Design review of the part shown in the three views and the two pictorial views. Dimensions are in mm from the part's minimum x, y and z. Round coordinates to 2 decimals unless told otherwise and drop trailing zeros. Loops run counter-clockwise (first coordinate to the right, second up) from the corner with the lowest first, then second, coordinate; pieces in that order, holes last. Notation, with made-up numbers: (49, 15) - (86, 15) arc R11 cw to (86, 36) - close; hole circle Ø3 at (74.25, 47.25). An arc over 180 degrees is marked (long way). Return JSON: item names as keys, results as strings. Group by question number.
(1) We need section B-B, the plane x = 60. Write out the cut boundary in (y, z), and give its area (3 significant figures).
(2) We need section A-A, the plane y = 40. Write out the cut boundary in (x, z), and give its area (3 significant figures).
(3) Clearance check with flat-ended pins moving along their axes: pin 1 (4 mm diameter, centred on x = 85, z = 309, fed in from +Y); pin 2 (12 mm diameter, centred on x = 85.5, z = 232.5, fed in from -Y); pin 3 (1.5 mm diameter, centred on y = 66.5, z = 629, fed in from +X). State where each tip first meets the part, or that it passes through.
(4) Wall thickness on L1, parallel to Z at x = 23, y = 36; L2, parallel to X at y = 38, z = 379; L3, parallel to X at y = 53, z = 588.5: over which ranges is each line inside the solid? List them lowest first. Write a range as [from, to].
(5) We need section C-C, the plane z = 817.5. Write out the cut boundary in (x, y).
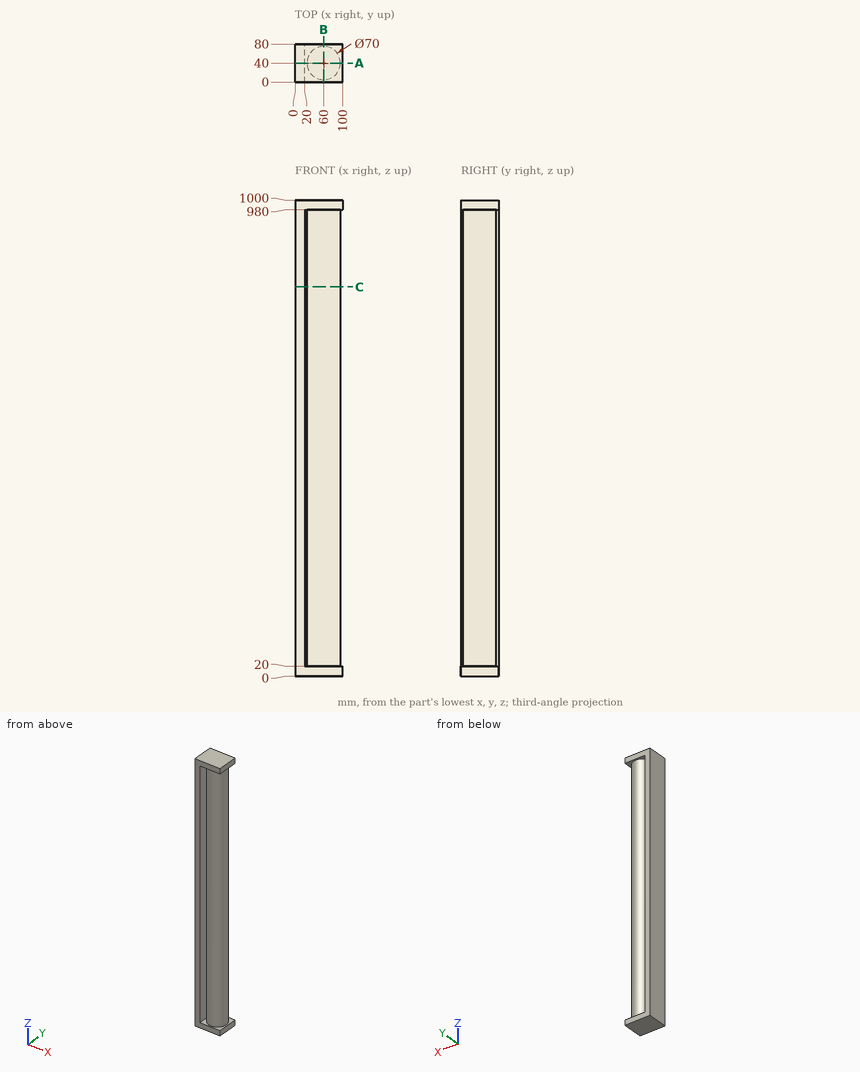
Solutions:
{
 "1": {"outline": "(0, 0) - (80, 0) - (80, 20) - (75, 20) - (75, 980) - (80, 980) - (80, 1000) - (0, 1000) - (0, 980) - (5, 980) - (5, 20) - (0, 20) - close", "area": "70,400 mm^2"},
 "2": {"outline": "(0, 0) - (100, 0) - (100, 20) - (95, 20) - (95, 980) - (100, 980) - (100, 1000) - (0, 1000) - close; hole (20, 20) - (25, 20) - (25, 980) - (20, 980) - close", "area": "90,400 mm^2"},
 "3": {"pin 1": "y = 66.38", "pin 2": "y = 10.94", "pin 3": "x = 83.71"},
 "4": {"L1": "[0, 20], [980, 1000]", "L2": "[0, 20], [25.06, 94.94]", "L3": "[0, 20], [27.5, 92.5]"},
 "5": {"outline": "(0, 0) - (20, 0) - (20, 80) - (0, 80) - close; circle Ø70 at (60, 40)"}
}
